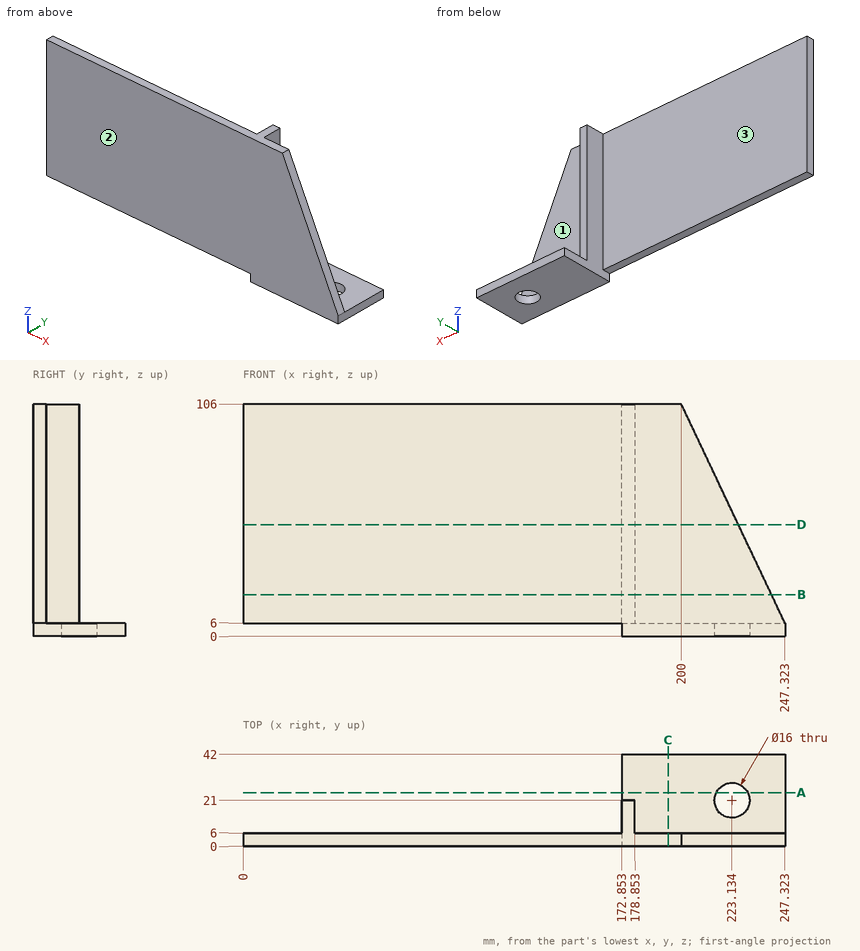
The drawing under review shows one solid part. Ordinate dimensions are in mm from its lowest x, y, z. A direction names the side the tool comes from. Round coordinates to 2 decimals unless told otherwise and drop trailing zeros. Write each loop counter-clockwise with the first axis right and the second up, starting at its lowest first coordinate (ties: lowest second). Pieces come first, ordered by that corner, then holes.
(1) Insertion check: pin 1 (3 mm diameter, centred on x = 211.5, z = 75.5, fed in from +Y); pin 2 (6.5 mm diameter, centred on x = 177.5, z = 59.5, fed in from +Y); pin 3 (5 mm diameter, centred on x = 73, y = 4.5, fed in from -Z). Each pin has a flat end and moves straight along its axis. Give the tip position at first contact, or say it passes through.
(2) We need section A-A on y = 24.5. Give the boundary of the cut face in (x, z).
(3) We need section B-B on z = 19. Give the boundary of the cut face in (x, y).
(4) Wall thickness on L1, parallel to Z at x = 178, y = 34; L2, parallel to X at y = 10, z = 86: over which ranges is each line inside the solid? List them lowest first.
(5) We need section C-C on x = 194. Give the boundary of the cut face in (y, z), and give its area (3 significant figures).
(6) Machinability: for the marked faces 1, 2 and 3, which of the approach directions +Z, -Z, +X, -X, +Y, -Y give a long, thin tool a straight path to every point of the face, cutting with its end or side? Answer none if there is none.
(7) We need section D-D on z = 51. Give the boundary of the cut face in (x, y), and give its area (3 significant figures).
Findings below:
1. pin 1: stops at y = 6
1. pin 2: stops at y = 21
1. pin 3: stops at z = 6
2. outline: (172.85, 0) - (215.94, 0) - (215.94, 6) - (172.85, 6) - close; (230.33, 0) - (247.32, 0) - (247.32, 6) - (230.33, 6) - close
3. outline: (0, 0) - (241.17, 0) - (241.17, 6) - (178.85, 6) - (178.85, 21) - (172.85, 21) - (172.85, 6) - (0, 6) - close
4. L1: z = 0 to 6
4. L2: x = 172.85 to 178.85
5. outline: (0, 0) - (42, 0) - (42, 6) - (6, 6) - (6, 106) - (0, 106) - close
5. area: 852 mm2
6. face 1: +Z, +X, +Y
6. face 2: +Z, -Z, +X, -X, -Y
6. face 3: +Z, -Z, -X, +Y
7. outline: (0, 0) - (226.03, 0) - (226.03, 6) - (178.85, 6) - (178.85, 21) - (172.85, 21) - (172.85, 6) - (0, 6) - close
7. area: 1,450 mm2
